The listing builds one solid part. Answer for the finished solid, in the listing's coordinates (mm). A direction names the side the tool comes from. Round coordinates to 2 decimals unless told otherwise and drop trailing zeros. Loops run counter-clockwise (first coordinate to the right, second up) from the corner with the lowest first, then second, coordinate; pieces in that order, holes last. Notation, with made-up numbers: (-28, 87.5) - (11, 87.5) arc R4 cw to (11, 93.5) - close; hole circle Ø10 at (34.5, 47). An arc over 180 degrees is marked (long way). Write item = value, one per line. Start each with the question number.
1) Straight lines are drawn through the part: line 1 along Y through (x, z) = (150.5, -108); line 2 along Z through (x, y) = (65, -349); line 3 along Z through (x, y) = (54, 475). For each, find the intervals that lie inside material, in ascending order.
2) A tool of negligible diameter and unlimited length cuts with its end or side. For faces 1 (the flat face through (78, 11, -577.5)), 2 (the flat face through (78, -459, 87)), 3 (the flat face through (78, -520, -236)), from which of +Z, -Z, +X, -X, +Y, -Y can it reach the whole face along a straight path? Write none if from no direction.
3) Section B-B, the plane y = 475 is taken. Determine the outline of the cut face in (x, z), and give its area (3 significant figures).
4) Given pin 1 Ø8 at (x, y) = (61, -143) entering from +Z; pin 2 Ø2 at (x, y) = (92.5, 287) entering from -Z; pin 3 Ø6 at (x, z) = (120, 21.5) entering from -Y, each flat-ended and moving along its own axis, determine where each tip first touches the part or whether it passes through.
5) Section D-D, the plane y = 21 is taken. Determine the outline of the cut face in (x, z), and give its area (3 significant figures).
6) For a pull along Z with two mould halves and no side action, classify faces 4 (the flat face through (159, -460, -233)), 5 (the flat face through (78.387, -496.324, 310.28)), 6 (the cylindrical face through (78.387, 467.491, -553.654)) as released by +Z, released by -Z, zero draft, split by the parting line, or undercut.
7) Section C-C, the plane z = -28.5 is taken. Determine the outline of the cut face in (x, y), and give its area (3 significant figures).
from build123d import *

# Parameters (mm, degrees)
SKETCH1_R           = 25
BOSS_EXTRUDE1_DEPTH = 159
FILLET1_R           = 60
FILLET2_R           = 60
FILLET3_R           = 100
FILLET4_R           = 6.498072


with BuildPart() as part:
    # Sketch1 → Boss-Extrude1 (new body)
    with BuildSketch(Plane(origin=(0, 0, 0), x_dir=(0, 0, -1), z_dir=(1, 0, 0))):
        with BuildLine():
            Line((577.5, 430), (577.5, -520))
            Line((577.5, -520), (-12.5, -520))
            Line((-12.5, -520), (-622.5, -471.5))
            Line((-622.5, -471.5), (-622.5, -459))
            Line((-622.5, -459), (516.5, -459))
            Line((516.5, -459), (516.5, 430))
            Line((516.5, 430), (516.5, 520))
            Line((516.5, 520), (577.5, 520))
            ThreePointArc((577.5, 520), (622.5, 475), (577.5, 430))
        make_face()
        with Locations(Location((577.5, 475, 0), (0, 0, 180))):
            Circle(SKETCH1_R, mode=Mode.SUBTRACT)
    extrude(amount=BOSS_EXTRUDE1_DEPTH)

    # Fillet1
    fillet1_edges = [part.edges().sort_by_distance(p)[0] for p in [
        (79.5, 520, -516.5),
    ]]
    fillet(fillet1_edges, radius=FILLET1_R)

    # Fillet2
    fillet2_edges = [part.edges().sort_by_distance(p)[0] for p in [
        (79.5, -459, -516.5),
    ]]
    fillet(fillet2_edges, radius=FILLET2_R)

    # Fillet3
    fillet3_edges = [part.edges().sort_by_distance(p)[0] for p in [
        (79.5, -520, -577.5),
    ]]
    fillet(fillet3_edges, radius=FILLET3_R)

    # Fillet4
    fillet4_edges = [part.edges().sort_by_distance(p)[0] for p in [
        (79.5, -471.5, 622.5),
        (79.5, -459, 622.5),
    ]]
    fillet(fillet4_edges, radius=FILLET4_R - 0.0001)  # a hair under: the kernel refuses the full size


solid = part.part
Geometry check:
q1.line_1 = -520 to -459
q1.line_2 = -577.5 to -516.5
q1.line_3 = -622.5 to -602.5, -552.5 to -518.41
q2.face_1 = -Z, +X, -X, -Y
q2.face_2 = +Z, +X, -X, +Y
q2.face_3 = +Z, -Z, +X, -X, -Y
q3.outline = (0, -622.5) - (159, -622.5) - (159, -602.5) - (0, -602.5) - close; (0, -552.5) - (159, -552.5) - (159, -518.41) - (0, -518.41) - close
q3.area = 8,600 mm2
q4.pin_1 = -516.5
q4.pin_2 = -577.5
q4.pin_3 = -519.52
q5.outline = (0, -577.5) - (159, -577.5) - (159, -516.5) - (0, -516.5) - close
q5.area = 9,700 mm2
q6.face_4 = zero draft
q6.face_5 = released by +Z
q6.face_6 = undercut
q7.outline = (0, -520) - (159, -520) - (159, -459) - (0, -459) - close
q7.area = 9,700 mm2
